Design review of the part built by this model. Coordinates are the model's own, in mm. A direction names the side the tool comes from. Give positions to 0.01 mm unless a question says otherwise; leave off trailing zeros. Loops run counter-clockwise (first coordinate to the right, second up) from the corner with the lowest first, then second, coordinate; pieces in that order, holes last. Notation, with made-up numbers: (-10, -27.75) -> (43, -27.75) arc R14 cw to (43, -0.75) -> close; hole circle Ø3 at (-14, -10). An arc over 180 degrees is marked (long way). Answer in a Markdown table with one row per item. Add a question column.
(1) For line 1 (Z direction, x = -19, y = -17) (3 decimals); line 2 (Z direction, x = 119.5, y = -24.5); line 3 (X direction, y = -2, z = -3.5) (3 decimals), list the stretches that pass through material, from the lowest coordinate up.
(2) Consider section B-B on x = 61. Write out the cut boundary in (y, z), then the cut area to 3 significant figures.
(3) For faces 4 (the flat face through (1, -36, 9.525)), 5 (the flat face through (94, 0, 57.855)), 6 (the flat face through (1, 35, 9.525)), 7 (the flat face through (64, -25.4, 66)), list the 3-axis set-ups (+Z, -Z, +X, -X, +Y, -Y) from which the entire face can be reached by the end or side of a thin tool; tool diameter is ignored.
(4) Consider section C-C on z = 5.5. Write out the cut boundary in (x, y) (3 decimals), then the cut area to 3 significant figures.
(5) For pin 1 (11.5 mm diameter, centred on x = 72.5, y = -3.5, fed in from +Z); pin 2 (5 mm diameter, centred on y = 13.5, z = 31, fed in from -X) (3 decimals); pin 3 (16.5 mm diameter, centred on x = -12.5, y = 23, fed in from +Z) (3 decimals), all flat-tipped, find the tip position at first contact; note any pin that passes through.
(6) Draft analysis for pull direction X (two halves, no side actions). For faces 1 (the flat face through (-4, 7.938, 38)), 2 (the flat face through (69, 0, 76.905)), 3 (the flat face through (22.225, -17, 26)), state which applies: +X half, -X half, draft (parallel to the pull), parting line (faces both ways), or undercut.
(7) Consider section A-A on y = -11. Write out the cut boundary in (x, z) (3 decimals).
from build123d import *

# Parameters (mm, degrees)
F1_DEPTH = 63.5
F2_DEPTH = 25.4
F3_DEPTH = 25.4
F4_DEPTH = 7.9375


with BuildPart() as f1:
    # F0 (on Front) → F1 (new body, symmetric)
    with BuildSketch(Plane.XZ):
        Polygon((41.275, -9.525), (41.275, 9.525), (22.225, 9.525), (-41.275, 9.525), (-41.275, -9.525), align=None)
    extrude(amount=F1_DEPTH, both=True)

    # F0 (on Front) → F2 (join, symmetric)
    with BuildSketch(Plane.XZ):
        with BuildLine():
            Line((22.225, 9.525), (41.275, 9.525))
            Line((41.275, 9.525), (41.275, 41.979897))
            ThreePointArc((41.275, 41.979897), (45.92468, 53.205217), (57.15, 57.854897))
            Line((57.15, 57.854897), (80.508934, 57.854897))
            Line((80.508934, 57.854897), (80.508934, 76.904897))
            Line((80.508934, 76.904897), (57.15, 76.904897))
            ThreePointArc((57.15, 76.904897), (32.454296, 66.675601), (22.225, 41.979897))
            Line((22.225, 41.979897), (22.225, 9.525))
        make_face()
    extrude(amount=F2_DEPTH, both=True)

    # F0 (on Front) → F3 (join, symmetric)
    with BuildSketch(Plane.XZ):
        Polygon((80.508934, 76.904897), (80.508934, 57.854897), (131.308934, 57.854897), (131.308934, 86.429897), (80.508934, 86.429897), align=None)
    extrude(amount=F3_DEPTH, both=True)

    # F0 (on Front) → F4 (join, symmetric)
    with BuildSketch(Plane.XZ):
        with BuildLine():
            Line((-41.275, 9.525), (22.225, 9.525))
            Line((22.225, 9.525), (22.225, 41.979897))
            ThreePointArc((22.225, 41.979897), (32.454296, 66.675601), (57.15, 76.904897))
            add(Edge.make_bspline(
                [(-41.275, 9.525), (-42.17181, 43.657206), (19.351373, 81.069473), (57.15, 76.904897)],
                knots=[0, 0, 0, 0, 119.279215, 119.279215, 119.279215, 119.279215], degree=3))
        make_face()
    extrude(amount=F4_DEPTH, both=True)


solid = f1.part
Values follow:
| question | item | result |
|---|---|---|
| 1 | line 1 | -9.525 to 9.525 |
| 1 | line 2 | 57.85 to 86.43 |
| 1 | line 3 | -41.275 to 41.275 |
| 2 | outline | (-25.4, 57.85) -> (25.4, 57.85) -> (25.4, 76.9) -> (-25.4, 76.9) -> close |
| 2 | area | 968 mm2 |
| 3 | face 4 | +Z, -X, -Y |
| 3 | face 5 | -Z, +X, +Y, -Y |
| 3 | face 6 | +Z, -X, +Y |
| 3 | face 7 | +Z, +X, -X, -Y |
| 4 | outline | (-41.275, -63.5) -> (41.275, -63.5) -> (41.275, 63.5) -> (-41.275, 63.5) -> close |
| 4 | area | 10,500 mm2 |
| 5 | pin 1 | z = 76.9 |
| 5 | pin 2 | x = 22.225 |
| 5 | pin 3 | z = 9.525 |
| 6 | face 1 | draft |
| 6 | face 2 | undercut |
| 6 | face 3 | -X half |
| 7 | outline | (-41.275, -9.525) -> (41.275, -9.525) -> (41.275, 41.98) arc R15.875 cw to (57.15, 57.855) -> (131.309, 57.855) -> (131.309, 86.43) -> (80.509, 86.43) -> (80.509, 76.905) -> (57.15, 76.905) arc R34.925 ccw to (22.225, 41.98) -> (22.225, 9.525) -> (-41.275, 9.525) -> close |
